Build history of the part. All positions in model axes, mm. Face numbers are marked on the shaded views. A direction names the side the tool comes from. Round coordinates to 2 decimals unless told otherwise and drop trailing zeros. Order: outer loops, then holes, each group sorted by start corner. A loop starts at its lowest first (then second) coordinate and runs counter-clockwise, first axis right, second up. Notation, with made-up numbers: M 17,-29.5 L 43,-29.5 A20 cw 43,-5.5 Z; hole C 84.25,65.5 d9. An arc over 180 degrees is marked long. Use CSV: the item, a comma, the result in double quotes.
from build123d import *

# Parameters (mm, degrees)
SKETCH4_R          = 11.782777778
SKETCH4_R_2        = 8.480777778
CUT_EXTRUDE2_DEPTH = 1.27
SKETCH5_R          = 6.096
CUT_EXTRUDE3_DEPTH = 0.635


with BuildPart() as part:
    # Sketch1 → Revolve1 (revolve)
    with BuildSketch(Plane.XY, mode=Mode.PRIVATE) as revolve1_sk:
        with BuildLine():
            Line((5.291666667, 22.225), (6.614583333, 22.225))
            Line((6.614583333, 22.225), (6.614583333, 9.877777778))
            Line((6.614583333, 9.877777778), (7.9375, 9.877777778))
            Line((7.9375, 9.877777778), (7.9375, 3.175))
            Line((7.9375, 3.175), (-7.9375, 3.175))
            Line((-7.9375, 3.175), (-7.9375, 9.877777778))
            Line((-7.9375, 9.877777778), (-6.614583333, 9.877777778))
            Line((-6.614583333, 9.877777778), (-6.614583333, 22.225))
            Line((-6.614583333, 22.225), (-5.291666667, 22.225))
            Line((-5.291666667, 22.225), (-3.037856108, 19.544099682))
            ThreePointArc((-3.037856108, 19.544099682), (0, 18.12925), (3.037856108, 19.544099682))
            Line((3.037856108, 19.544099682), (5.291666667, 22.225))
        make_face()
    revolve(revolve1_sk.sketch.rotate(Axis((-7.9375, 0, 0), (1, 0, 0)), 90), axis=Axis((-7.9375, 0, 0), (1, 0, 0)))

    # Sketch2 → Cut-Revolve1 (revolve, cut)
    with BuildSketch(Plane.XY, mode=Mode.PRIVATE) as cut_revolve1_sk:
        Polygon((-7.9375, 9.877777778), (-6.614583333, 9.877777778), (-1.5875, 10.764188204), (-1.5875, 13.87175685), (-7.9375, 21.425061163), align=None)
        Polygon((7.9375, 9.877777778), (7.9375, 21.425061163), (1.5875, 13.87175685), (1.5875, 10.764188204), (6.614583333, 9.877777778), align=None)
    revolve(cut_revolve1_sk.sketch.rotate(Axis((-7.9375, 0, 0), (1, 0, 0)), 90), axis=Axis((-7.9375, 0, 0), (1, 0, 0)), mode=Mode.SUBTRACT)

    # Sketch4 → Cut-Extrude2 (cut)
    with BuildSketch(Plane.ZY.offset(7.9375)):
        Circle(SKETCH4_R)
        Circle(SKETCH4_R_2, mode=Mode.SUBTRACT)
    cut_extrude2 = extrude(amount=-CUT_EXTRUDE2_DEPTH, mode=Mode.SUBTRACT)

    # Sketch5 → Cut-Extrude3 (cut)
    with BuildSketch(Plane.ZY.offset(7.9375)):
        Circle(SKETCH5_R)
    cut_extrude3 = extrude(amount=-CUT_EXTRUDE3_DEPTH, mode=Mode.SUBTRACT)

    # Mirror1: Cut-Extrude2, Cut-Extrude3 across plane
    add(cut_extrude2.mirror(Plane(origin=(0, 0, 0), x_dir=(0, 0, 1), z_dir=(1, 0, 0))), mode=Mode.SUBTRACT)
    add(cut_extrude3.mirror(Plane(origin=(0, 0, 0), x_dir=(0, 0, 1), z_dir=(1, 0, 0))), mode=Mode.SUBTRACT)


solid = part.part
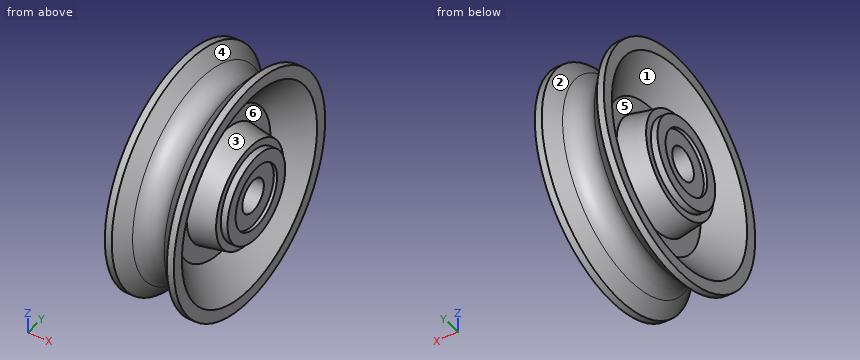
(1) Wall check: line 1 (Y direction, x = 7.6, z = 0); line 2 (Z direction, x = -5, y = 0.5); line 3 (Z direction, x = -5.5, y = -9). Give the ranges that are in metal, low to high. Write a range as from..to.
Answer block:
line 1,"y = -8.48..-6.1, 6.1..8.48"
line 2,"z = -21.87..-17.92, -10.15..-3.14, 3.14..10.15, 17.92..21.87"
line 3,"z = -20.32..-16.19, -4.53..4.53, 16.19..20.32"
(2) Cut at C-C, the plane x = 4.75. Give the cut face in (y, z) (3 decimals), and give its area (3 significant figures).
Answer block:
outline,"C 0,0 d43.161; C 0,0 d20.413; hole C 0,0 d35.267; hole C 0,0 d6.35"
area,"782 mm²"
(3) Drop flat-ended pins along their axis: pin 1 (16 mm diameter, centred on y = 4, z = -4.5, fed in from +X); pin 2 (6 mm diameter, centred on x = -4.5, y = -12.5, fed in from +Z); pin 3 (2 mm diameter, centred on x = 6, y = -13, fed in from -Z); pin 4 (3.5 mm diameter, centred on y = 1.5, z = -2.5, fed in from +X). Give the stop position or say it passes through.
Answer block:
pin 1,"stops at x = 7.94"
pin 2,"stops at z = 20.04"
pin 3,"stops at z = -18.71"
pin 4,"stops at x = 7.3"
(4) Two-plate mould, pull along X, no slides. Class the marked faces 1, 2 and 3: released by +X, released by -X, zero draft, split by the parting line, or undercut.
Answer block:
face 1,"released by -X"
face 2,"undercut"
face 3,"released by +X"
(5) Cut at B-B, the plane x = -1. Give the cut face in (y, z) (3 decimals).
Answer block:
outline,"C 0,0 d36.515; hole C 0,0 d6.35"
(6) Tool access for the marked faces 4, 5 and 6: list every direction of +Z, -Z, +X, -X, +Y, -Y with a clear straight run to the whole face (end or side of a thin tool).
Answer block:
face 4,"none"
face 5,"-X"
face 6,"+X"
(7) Cut at A-A, the plane x = 2.25. Give the cut face in (y, z) (3 decimals).
Answer block:
outline,"C 0,0 d37.657; C 0,0 d21.295; hole C 0,0 d29.32; hole C 0,0 d6.35"
